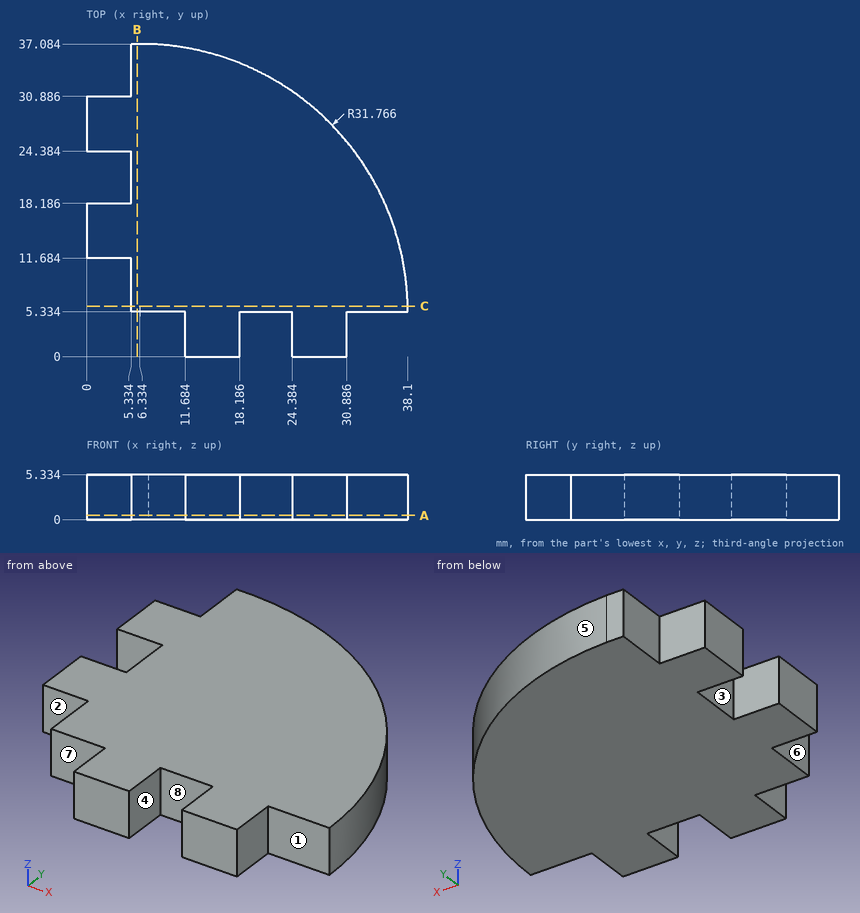
Verification items for this drawing (mm, ordinates from the low corner). A direction names the side the tool comes from. Give positions to 0.01 mm unless a question says otherwise; leave off trailing zeros. Loops run counter-clockwise (first coordinate to the right, second up) from the corner with the lowest first, then second, coordinate; pieces in that order, holes last. Notation, with made-up numbers: M 0,-14 L 47,-14 A29 ccw 47,14 Z; hole C 9.25,82.5 d4. An arc over 180 degrees is marked long. Write item = value, one per line. Start each with the question number.
1. Section check C-C, the plane y = 6. Enter the section's corners in (x, z).
2. Go/stop test with flat-tipped pins: P1, Ø1.6, axis at x = 3.5, z = 2, coming from the -Y side; P2, Ø1.6, axis at y = 3.5, z = 2, coming from the +X side; P3, Ø1.6, axis at x = 9, z = 1.5, coming from the -Y side; P4, Ø1.5, axis at x = 33, y = 25.5, coming from the +Z side. Record where each tip stops, or that it passes through.
3. Section check A-A, the plane z = 0.5. Enter the section's corners in (x, y) (1 decimal).
4. Section check B-B, the plane x = 6. Enter the section's corners in (y, z).
5. Thickness scan on probe 1 along Y at (x, z) = (4.5, 0.95); probe 2 along X at (y, z) = (6, 2.65). Record the ranges inside material, lowest first.
6. Draft check along X on the marked faces 5, 6, 7 and 8. Enter one of: +X half, -X half, draft (parallel to the pull), parting line (faces both ways), or undercut.
7. Tool access check on the marked faces 1, 2, 3 and 4. Record the directions out of +Z, -Z, +X, -X, +Y, -Y that give a thin tool (end or side, any length) a straight path to the whole face; none if there is none.
Values follow:
q1.outline = M 5.33,0 L 38.09,0 L 38.09,5.33 L 5.33,5.33 Z
q2.P1 = 11.68
q2.P2 = 30.89
q2.P3 = 5.33
q2.P4 = through
q3.outline = M 0,11.7 L 5.3,11.7 L 5.3,5.3 L 11.7,5.3 L 11.7,0 L 18.2,0 L 18.2,5.3 L 24.4,5.3 L 24.4,0 L 30.9,0 L 30.9,5.3 L 38.1,5.3 A31.8 ccw 7.3,37.1 L 5.3,37.1 L 5.3,30.9 L 0,30.9 L 0,24.4 L 5.3,24.4 L 5.3,18.2 L 0,18.2 Z
q4.outline = M 5.33,0 L 37.08,0 L 37.08,5.33 L 5.33,5.33 Z
q5.probe_1 = 11.68 to 18.19, 24.38 to 30.89
q5.probe_2 = 5.33 to 38.09
q6.face_5 = +X half
q6.face_6 = -X half
q6.face_7 = draft
q6.face_8 = undercut
q7.face_1 = +Z, -Z, +X, -Y
q7.face_2 = +Z, -Z, -X, -Y
q7.face_3 = +Z, -Z, -X
q7.face_4 = +Z, -Z, -Y
